from build123d import *

# Parameters (mm, degrees)
SKETCH_1_R      = 1.3
EXTRUDE_1_DEPTH = 2


with BuildPart() as part:
    # 草图1 → 凸台-拉伸1 (new body)
    with BuildSketch(Plane.XY):
        with BuildLine():
            Line((-1, 3.5), (50, 3.5))
            ThreePointArc((50, 3.5), (51.767766953, 2.767766953), (52.5, 1))
            Line((52.5, 1), (52.5, -79))
            ThreePointArc((52.5, -79), (51.767766953, -80.767766953), (50, -81.5))
            Line((50, -81.5), (-1, -81.5))
            ThreePointArc((-1, -81.5), (-2.767766953, -80.767766953), (-3.5, -79))
            Line((-3.5, -79), (-3.5, 1))
            ThreePointArc((-3.5, 1), (-2.767766953, 2.767766953), (-1, 3.5))
        make_face()
        with Locations((49, 0)):
            Circle(SKETCH_1_R, mode=Mode.SUBTRACT)
        with Locations((49, -58)):
            Circle(SKETCH_1_R, mode=Mode.SUBTRACT)
        with Locations((0, -58)):
            Circle(SKETCH_1_R, mode=Mode.SUBTRACT)
        Circle(SKETCH_1_R, mode=Mode.SUBTRACT)
    extrude(amount=EXTRUDE_1_DEPTH)


solid = part.part
Design review of the part built by this model. Coordinates are the model's own, in mm. Round coordinates to 2 decimals unless told otherwise and drop trailing zeros. Loops run counter-clockwise (first coordinate to the right, second up) from the corner with the lowest first, then second, coordinate; pieces in that order, holes last. Notation, with made-up numbers: (29, -37) -> (34, -37) arc R31 ccw to (34, -1) -> close; hole circle Ø1 at (85, 79.25). An arc over 180 degrees is marked (long way). Use one line per item in the form item = value. Start each with the question number.
Q1. Draft analysis for pull direction Y (two halves, no side actions). For faces 1 (the face through (24, 3.5, 1)), 2 (the face through (25, -81.5, 1)), 3 (the face through (47.7, 0.06, 0.99)), state which applies: +Y half, -Y half, draft (parallel to the pull), parting line (faces both ways), or undercut.
Q2. We need section A-A on y = -58. Give the boundary of the cut face in (x, z).
Q3. We need section B-B on x = 49. Give the boundary of the cut face in (y, z), then the cut area to 3 significant figures.
Q4. For pin 1 Ø2.5 at (x, y) = (0, -58) entering from -Z, flat-tipped, find the tip position at first contact; note if it passes through.
Q5. Wall thickness on line 1 along Y through (x, z) = (49, 0.8); line 2 along Y through (x, z) = (48, 1.1): over which ranges is each line inside the solid? List them lowest first. Write a range as [from, to].
Calculated:
q1.face_1 = +Y half
q1.face_2 = -Y half
q1.face_3 = undercut
q2.outline = (-3.5, 0) -> (-1.3, 0) -> (-1.3, 2) -> (-3.5, 2) -> close; (1.3, 0) -> (47.7, 0) -> (47.7, 2) -> (1.3, 2) -> close; (50.3, 0) -> (52.5, 0) -> (52.5, 2) -> (50.3, 2) -> close
q3.outline = (-81.5, 0) -> (-59.3, 0) -> (-59.3, 2) -> (-81.5, 2) -> close; (-56.7, 0) -> (-1.3, 0) -> (-1.3, 2) -> (-56.7, 2) -> close; (1.3, 0) -> (3.5, 0) -> (3.5, 2) -> (1.3, 2) -> close
q3.area = 160 mm²
q4.pin_1 = through
q5.line_1 = [-81.5, -59.3], [-56.7, -1.3], [1.3, 3.5]
q5.line_2 = [-81.5, -58.83], [-57.17, -0.83], [0.83, 3.5]
